Here's how the part is built. I have some questions about the finished solid (model axes, mm). Round coordinates to 2 decimals unless told otherwise and drop trailing zeros. Write each loop counter-clockwise with the first axis right and the second up, starting at its lowest first coordinate (ties: lowest second). Pieces come first, ordered by that corner, then holes. Notation, with made-up numbers: (35, 12) -> (91, 12) arc R21 ccw to (91, 43) -> close; hole circle Ø5 at (0.5, -20). An arc over 180 degrees is marked (long way). Put each result on its own line as item: value. Start each with the question number.
1. Suppose I cut it at B-B (z = 3.5). Please give me the cut outline in (x, y) (3 decimals), then the cut area to 3 significant figures.
2. For pin 1 (3 mm diameter, centred on y = -2, z = -1.5, fed in from -X); pin 2 (1.5 mm diameter, centred on y = -4, z = 2.5, fed in from -X); pin 3 (1 mm diameter, centred on x = -0.5, y = 2, fed in from +Z); pin 4 (2 mm diameter, centred on y = -0.5, z = -0.5, fed in from -X), each with a flat end and sliding along its axis, tell me the tip position at first contact or that it passes through.
3. I need wall thicknesses on probe 1 along Y at (x, z) = (0, 1.5) (3 decimals); probe 2 along X at (y, z) = (1.25, 3.5); probe 3 along Y at (x, z) = (-1.75, 0.25) (3 decimals). Which ranges of each line are inside material? Lowest first, please. Write a range as from..to.
4. Suppose I cut it at A-A (z = 2.5). Please give me the cut outline in (x, y) (3 decimals).
5. We'd pull the mould along Y, two halves only. Please class faces 1 (the face through (7.435, -4.373, 0.063)), 2 (the face through (-0.59, 4.46, -0.06)), 3 (the face through (8.949, 0.022, -4.176)): +Y half, -Y half, draft (parallel to the pull), parting line (faces both ways), or undercut.
```python
from build123d import *

# Parameters (mm, degrees)
SKETCH4_R           = 4.5
BOSS_EXTRUDE2_DEPTH = 4.5
SKETCH5_OUTSIDE_W   = 45.486
SKETCH5_OUTSIDE_H   = 42.818
SKETCH5_OUTSIDE_R   = 8.625
CUT_EXTRUDE2_DEPTH  = 9
CUT_EXTRUDE2_TAPER  = 45


with BuildPart() as part:
    # Sketch4 → Boss-Extrude2 (new body, symmetric)
    with BuildSketch(Plane.XY):
        Polygon((9.959292144, 0), (4.979646072, 8.625), (-4.979646072, 8.625), (-9.959292144, 0), (-4.979646072, -8.625), (4.979646072, -8.625), align=None)
        Circle(SKETCH4_R, mode=Mode.SUBTRACT)
    extrude(amount=BOSS_EXTRUDE2_DEPTH, both=True)

    # Sketch5 outside → Cut-Extrude2 (cut)
    with BuildSketch(Plane.XY.offset(4.5)):
        Rectangle(SKETCH5_OUTSIDE_W, SKETCH5_OUTSIDE_H)
        Circle(SKETCH5_OUTSIDE_R, mode=Mode.SUBTRACT)
    cut_extrude2 = extrude(amount=-CUT_EXTRUDE2_DEPTH, taper=CUT_EXTRUDE2_TAPER, mode=Mode.SUBTRACT)

    # Mirror1: Cut-Extrude2 across plane
    add(cut_extrude2.mirror(Plane.XY), mode=Mode.SUBTRACT)


solid = part.part
```
Verdict:
1. outline: (-9.605, -0.613) -> (-5.333, -8.012) arc R9.625 ccw to (-4.272, -8.625) -> (4.272, -8.625) arc R9.625 ccw to (5.333, -8.012) -> (9.605, -0.613) arc R9.625 ccw to (9.605, 0.613) -> (5.333, 8.012) arc R9.625 ccw to (4.272, 8.625) -> (-4.272, 8.625) arc R9.625 ccw to (-5.333, 8.012) -> (-9.605, 0.613) arc R9.625 ccw to start; hole circle Ø9 at (0, 0)
1. area: 193 mm^2
2. pin 1: stops at x = -9.67
2. pin 2: stops at x = -8.08
2. pin 3: passes through
2. pin 4: stops at x = -9.96
3. probe 1: y = -8.625..-4.5, 4.5..8.625
3. probe 2: x = -9.24..-4.32, 4.32..9.24
3. probe 3: y = -8.625..-4.146, 4.146..8.625
4. outline: (-9.959, 0) -> (-4.98, -8.625) -> (4.98, -8.625) -> (9.959, 0) -> (4.98, 8.625) -> (-4.98, 8.625) -> close; hole circle Ø9 at (0, 0)
5. face 1: -Y half
5. face 2: undercut
5. face 3: parting line
